Can you work these out from the model? Positions are in its coordinate system, mm. Give positions to 0.01 mm unless a question says otherwise; leave off trailing zeros. Write each loop counter-clockwise with the first axis right and the second up, starting at its lowest first coordinate (ties: lowest second). Pieces come first, ordered by that corner, then holes.
1. Suppose I cut it at A-A (x = 17). Please give me the cut outline in (y, z), and give its area (3 significant figures).
2. I'm going to push flat-ended pins straight in: pin 1 (0.9 mm diameter, centred on y = 2, z = -3, fed in from +X); pin 2 (1.5 mm diameter, centred on x = -110, y = 1, fed in from +Z); pin 3 (8 mm diameter, centred on x = 136.5, z = -41.5, fed in from -Y); pin 4 (1.5 mm diameter, centred on x = 179.5, y = 1, fed in from -Z). Where does each tip first touch, or does it pass through?
3. If I drill on probe 1 along Z at (x, y) = (-105.5, 2.75); probe 2 along X at (y, z) = (0.95, -13); probe 3 along Z at (x, y) = (-141, 0.2), over which ranges is the centre line in solid material (lowest first)?
4. Suppose I cut it at B-B (z = -56.5). Please give me the cut outline in (x, y), and give its area (3 significant figures).
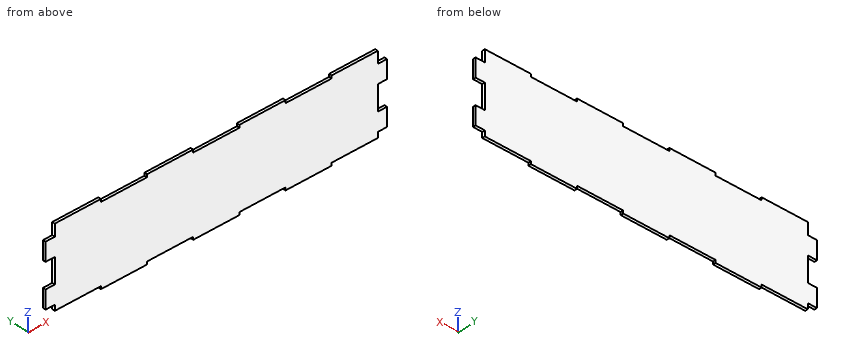
```python
from build123d import *

# Parameters (mm, degrees)
EXTRUDE_1_DEPTH = 3


with BuildPart() as part:
    # 스케치1 → 보스-돌출1 (new body)
    with BuildSketch(Plane(origin=(0, 0, 0), x_dir=(1, 0, 0), z_dir=(0, 1, 0))):
        Polygon((-175, 3.97), (-175, 13.97), (-185, 13.97), (-185, 33.97), (-175, 33.97), (-175, 61.2), (-185, 61.2), (-185, 81.2), (-175, 81.2), (-175, 87.23), (-125, 87.23), (-125, 90.23), (-75, 90.23), (-75, 87.23), (-25, 87.23), (-25, 90.23), (25, 90.23), (25, 87.23), (75, 87.23), (75, 90.23), (125, 90.23), (125, 87.23), (175, 87.23), (175, 81.2), (185, 81.2), (185, 61.2), (175, 61.2), (175, 33.97), (185, 33.97), (185, 13.97), (175, 13.97), (175, 3.97), (175, 0.97), (125, 0.97), (125, 3.97), (75, 3.97), (75, 0.97), (25, 0.97), (25, 3.97), (-25, 3.97), (-25, 0.97), (-75, 0.97), (-75, 3.97), (-125, 3.97), (-125, 0.97), (-175, 0.97), align=None)
    extrude(amount=EXTRUDE_1_DEPTH)


solid = part.part
```
Checks:
1. outline: (0, -90.23) - (3, -90.23) - (3, -3.97) - (0, -3.97) - close
1. area: 259 mm2
2. pin 1: stops at x = 175
2. pin 2: stops at z = -3.97
2. pin 3: stops at y = 0
2. pin 4: stops at z = -81.2
3. probe 1: z = -90.23 to -3.97
3. probe 2: x = -175 to 175
3. probe 3: z = -87.23 to -0.97
4. outline: (-175, 0) - (175, 0) - (175, 3) - (-175, 3) - close
4. area: 1,050 mm2
